Source: three-view drawing plus pictorial views. Frame: mm from the lowest corner of the part. A direction names the side the tool comes from. Coordinates: 2 decimals unless noted, no trailing zeros. Write each loop counter-clockwise with the first axis right and the second up, starting at its lowest first coordinate (ties: lowest second). Pieces come first, ordered by that corner, then holes. Notation, with made-up numbers: M 41.5,62.5 L 63.5,62.5 A32 ccw 63.5,96.5 Z; hole C -4.75,-30 d5. An arc over 180 degrees is marked long. Answer as a JSON object with one key per item and string values. Group by question number.
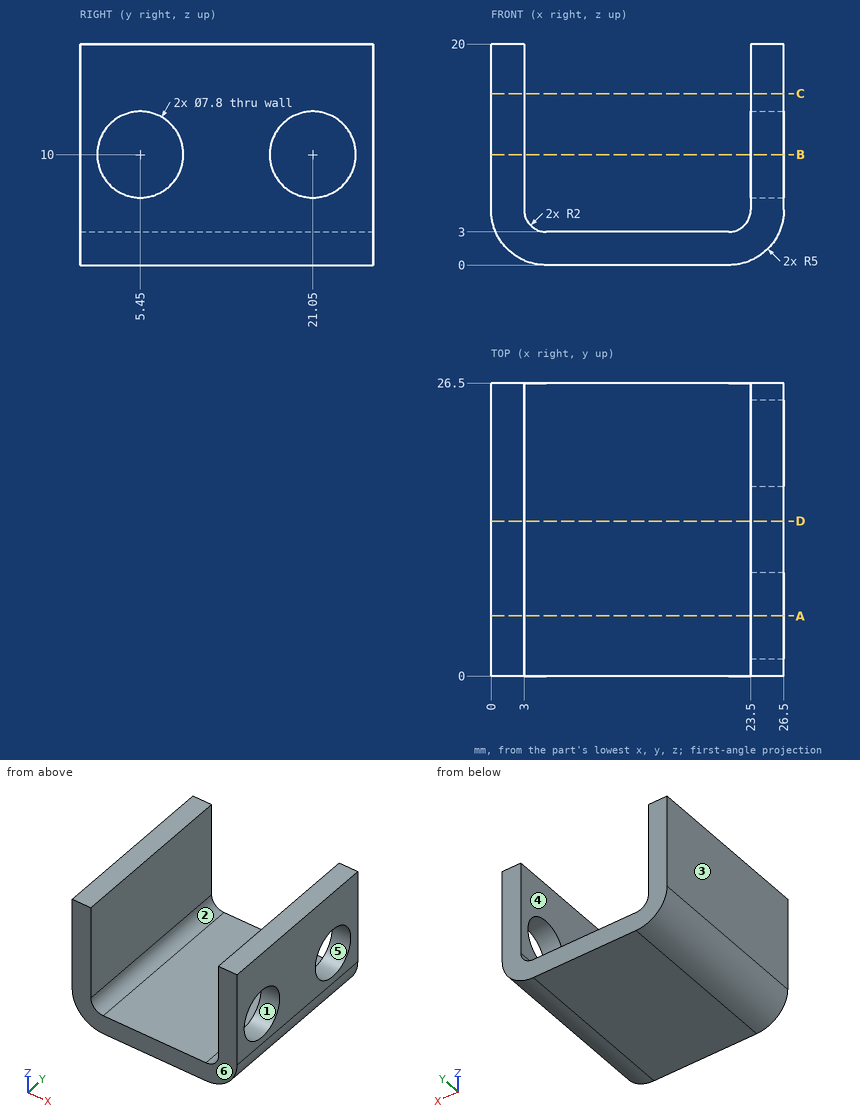
Q1. Section C-C, the plane z = 15.5. Return the cut outline in (x, y).
Q2. Pin query (flat end, axial travel): pin 1 Ø4 at (x, y) = (7.5, 9.5) entering from +Z. Return the tip coordinate at first contact, or that it passes through.
Q3. Section B-B, the plane z = 10. Return the cut outline in (x, y).
Q4. Access query for the marked faces 1, 2 and 3. Directions: +Z, -Z, +X, -X, +Y, -Y. A direction counts if a zero-diameter tool reaches every point of the face in a straight line with its end or side. Return the directions, or none.
Q5. Line query: line 1 (Y direction, x = 25, z = 11); line 2 (X direction, y = 24.25, z = 13.5); line 3 (Z direction, x = 20.5, y = 18.75). Output: solid intervals per line, ascending. Write a range as from..to.
Q6. Draft query along Y for the marked faces 4, 5 and 6. Return one class per face: released by +Y, released by -Y, zero draft, split by the parting line, or undercut.
Q7. Section D-D, the plane y = 14. Return the cut outline in (x, z).
Q8. Section A-A, the plane y = 5.45. Return the cut outline in (x, z).
Filled in:
{
 "1": {"outline": "M 0,0 L 3,0 L 3,26.5 L 0,26.5 Z; M 23.5,0 L 26.5,0 L 26.5,26.5 L 23.5,26.5 Z"},
 "2": {"pin 1": "z = 3"},
 "3": {"outline": "M 0,0 L 3,0 L 3,26.5 L 0,26.5 Z; M 23.5,0 L 26.5,0 L 26.5,1.55 L 23.5,1.55 Z; M 23.5,9.35 L 26.5,9.35 L 26.5,17.15 L 23.5,17.15 Z; M 23.5,24.95 L 26.5,24.95 L 26.5,26.5 L 23.5,26.5 Z"},
 "4": {"face 1": "+X", "face 2": "+Z, +Y, -Y", "face 3": "+Z, -Z, -X, +Y, -Y"},
 "5": {"line 1": "0..1.68, 9.22..17.28, 24.82..26.5", "line 2": "0..3, 23.5..26.5", "line 3": "0..3"},
 "6": {"face 4": "zero draft", "face 5": "undercut", "face 6": "released by -Y"},
 "7": {"outline": "M 0,5 A5 ccw 5,0 L 21.5,0 A5 ccw 26.5,5 L 26.5,20 L 23.5,20 L 23.5,5 A2 cw 21.5,3 L 5,3 A2 cw 3,5 L 3,20 L 0,20 Z"},
 "8": {"outline": "M 0,5 A5 ccw 5,0 L 21.5,0 A5 ccw 26.5,5 L 26.5,6.1 L 23.5,6.1 L 23.5,5 A2 cw 21.5,3 L 5,3 A2 cw 3,5 L 3,20 L 0,20 Z; M 23.5,13.9 L 26.5,13.9 L 26.5,20 L 23.5,20 Z"}
}
